from build123d import *

# Parameters (mm, degrees)
SKETCH1_W               = 13
SKETCH1_H               = 8
BOSS_EXTRUDE1_DEPTH     = 3
CUT_EXTRUDE1_DEPTH      = 16.556349186
CUT_EXTRUDE1_DEPTH_BACK = 16.556349186
CUT_EXTRUDE2_DEPTH      = 16.556349186
CUT_EXTRUDE2_DEPTH_BACK = 16.556349186
SKETCH4_R               = 1.8
CUT_EXTRUDE3_DEPTH      = 0.8
SKETCH5_W               = 8
SKETCH5_H               = 1
BOSS_EXTRUDE2_DEPTH     = 2
FILLET1_R               = 4
CUT_EXTRUDE4_DEPTH      = 0.4


with BuildPart() as part:
    # Sketch1 → Boss-Extrude1 (new body)
    with BuildSketch(Plane(origin=(0, 0, 0), x_dir=(1, 0, 0), z_dir=(0, 1, 0))):
        with Locations((6.5, 4)):
            Rectangle(SKETCH1_W, SKETCH1_H)
    extrude(amount=BOSS_EXTRUDE1_DEPTH)

    # Sketch2 → Cut-Extrude1 (cut, two sides: drawn at the far end of the back side and taken through both)
    with BuildSketch(Plane.XY.offset(-CUT_EXTRUDE1_DEPTH_BACK)):
        Polygon((0, 0), (0.6, 3), (0, 3), align=None)
        Polygon((13, 0), (12.4, 3), (13, 3), align=None)
    extrude(amount=CUT_EXTRUDE1_DEPTH + CUT_EXTRUDE1_DEPTH_BACK, mode=Mode.SUBTRACT)

    # Sketch3 → Cut-Extrude2 (cut, two sides: drawn at the far end of the back side and taken through both)
    with BuildSketch(Plane(origin=(0, 0, 0), x_dir=(0, 0, -1), z_dir=(1, 0, 0)).offset(-CUT_EXTRUDE2_DEPTH_BACK)):
        Polygon((0, 0), (0.6, 3), (0, 3), align=None)
        Polygon((8, 3), (7.4, 3), (8, 0), align=None)
    extrude(amount=CUT_EXTRUDE2_DEPTH + CUT_EXTRUDE2_DEPTH_BACK, mode=Mode.SUBTRACT)

    # Sketch4 → Cut-Extrude3 (cut)
    with BuildSketch(Plane.XZ):
        with Locations(Location((6.50000125, -3.75, 0), (0, 0, 270))):
            Circle(SKETCH4_R)
    extrude(amount=-CUT_EXTRUDE3_DEPTH, mode=Mode.SUBTRACT)

    # Sketch5 → Boss-Extrude2 (add)
    with BuildSketch(Plane.XZ):
        with Locations((6.500011, -7.5)):
            Rectangle(SKETCH5_W, SKETCH5_H)
    extrude(amount=BOSS_EXTRUDE2_DEPTH)

    # Fillet1
    # the kernel refuses this fillet: 4 mm, written as the material it takes off along each edge
    with BuildSketch(Plane(origin=(10.500011, -2, -16.660254038), x_dir=(0, 1, 0), z_dir=(0, 0, 1)), Plane(origin=(2.500011, -2, 1.660254038), x_dir=(0, 1, 0), z_dir=(0, 0, -1))) as fillet1_piece_1:
        with BuildLine():
            CenterArc((4, 3.464101615), FILLET1_R, 180, 60)
            Line((0, 3.464101615), (-0.08, 3.464101615))
            Line((-0.08, 3.464101615), (-0.08, 0))
            Line((-0.08, 0), (0, -0.08))
            ThreePointArc((0, -0.08), (1, -0.08), (1.96, -0.069282032))
            Line((1.96, -0.069282032), (2, 0))
        make_face()
    extrude(amount=18.320508076, mode=Mode.SUBTRACT)

    # Sketch6 → Cut-Extrude4 (cut)
    # profile 1 of 3: a face of its own
    with BuildSketch(Plane(origin=(0, 3, 0), x_dir=(1, 0, 0), z_dir=(0, 1, 0))):
        Polygon((5.356583629, 2.605681315), (4.744804782, 2.605681315), (4.491799975, 3.297989008), (3.340357667, 3.297989008), (3.087352859, 2.605681315), (2.471968244, 2.605681315), (3.605982667, 5.605681315), (4.217160552, 5.605681315), align=None)
        Polygon((4.308506705, 3.797989008), (3.914275936, 4.874912084), (3.52124709, 3.797989008), align=None, mode=Mode.SUBTRACT)
    # profile 2 of 3: a face of its own
    with BuildSketch(Plane(origin=(0, 3, 0), x_dir=(1, 0, 0), z_dir=(0, 1, 0))):
        Polygon((5.664275936, 2.605681315), (5.664275936, 5.605681315), (6.241199013, 5.605681315), (6.241199013, 3.105681315), (7.779660552, 3.105681315), (7.779660552, 2.605681315), align=None)
    # profile 3 of 3: a face of its own
    with BuildSketch(Plane(origin=(0, 3, 0), x_dir=(1, 0, 0), z_dir=(0, 1, 0))):
        Polygon((8.895045167, 2.605681315), (8.895045167, 5.105681315), (8.010429782, 5.105681315), (8.010429782, 5.605681315), (10.356583629, 5.605681315), (10.356583629, 5.105681315), (9.471968244, 5.105681315), (9.471968244, 2.605681315), align=None)
    extrude(amount=-CUT_EXTRUDE4_DEPTH, mode=Mode.SUBTRACT)


solid = part.part
For this review, take the finished solid that the model builds, in its own axes (mm). A direction names the side the tool comes from. Coordinates: 2 decimals unless noted, no trailing zeros. Loops run counter-clockwise (first coordinate to the right, second up) from the corner with the lowest first, then second, coordinate; pieces in that order, holes last. Notation, with made-up numbers: (67.5, 44) - (78.5, 44) arc R30 ccw to (78.5, 69) - close; hole circle Ø3 at (57.5, 20). An arc over 180 degrees is marked (long way). Return JSON: item names as keys, results as strings.
Item 1: Take a section at A-A (z = -5.25). Give the boundary of the cut face in (x, y).
Determined:
{"outline": "(0, 0) - (5.51, 0) - (5.51, 0.8) - (7.49, 0.8) - (7.49, 0) - (13, 0) - (12.4, 3) - (10.36, 3) - (10.36, 2.6) - (8.01, 2.6) - (8.01, 3) - (6.24, 3) - (6.24, 2.6) - (5.66, 2.6) - (5.66, 3) - (4.35, 3) - (4.35, 2.6) - (3.47, 2.6) - (3.47, 3) - (0.6, 3) - close"}
Item 2: For faces 1 (the flat face through (6.4, 1.5, -0.3)), 2 (the flat face through (7, 0.8, -4)), 3 (the flat face through (6, -1, -7)), 4 (the flat face through (4.779, 2.803, -4.127)), 5 (the flat face through (6.4, 1.5, -7.7)), list the 3-axis set-ups (+Z, -Z, +X, -X, +Y, -Y) from which the entire face can be reached by the end or side of a thin tool; tool diameter is ignored.
Determined:
{"face 1": "+Z, +X, -X, +Y", "face 2": "-Y", "face 3": "+Z, +X, -X, -Y", "face 4": "+Y", "face 5": "-Z, +X, -X, +Y"}
Item 3: Mouldability with a two-part tool opening along X and no side actions: class faces 6 (the flat face through (6, -1, -8)), 7 (the cylindrical face through (5.811, 0.394, -5.413)), 8 (the flat face through (0.3, 1.5, -4.1)) as pulls with the +X half, pulls with the -X half, needs draft (parallel to the pull), parting line crosses it, or undercut.
Determined:
{"face 6": "needs draft", "face 7": "undercut", "face 8": "pulls with the -X half"}
Item 4: Insertion check: pin 1 (3 mm diameter, centred on x = 8, z = -2.5, fed in from -Y); pin 2 (1.8 mm diameter, centred on x = 6, z = -4, fed in from -Y). Each pin has a flat end and moves straight along its axis. Give the tip position at first contact, or say it passes through.
Determined:
{"pin 1": "stops at y = 0", "pin 2": "stops at y = 0.8"}
Item 5: Take a section at B-B (x = 11). Give the boundary of the cut face in (y, z).
Determined:
{"outline": "(0, -8) - (3, -7.4) - (3, -0.6) - (0, 0) - close"}
Item 6: Take a section at C-C (y = -1.35). Give the boundary of the cut face in (x, z).
Determined:
{"outline": "(3.78, -8) - (9.22, -8) - (9.22, -7) - (3.78, -7) - close"}
Item 7: For line 1 (Y direction, x = 3.75, z = -0.75); line 2 (Z direction, x = 9.5, y = -0.05); line 3 (Z direction, x = 10.5, y = 0.7), list the stretches that pass through material, from the lowest coordinate up.
Determined:
{"line 1": "y = 0 to 3", "line 2": "z = -8 to -7", "line 3": "z = -7.86 to -0.14"}
Item 8: Take a section at D-D (x = 8.75). Give the boundary of the cut face in (y, z), then the cut area to 3 significant figures.
Determined:
{"outline": "(-1.61, -8) - (0, -8) - (3, -7.4) - (3, -5.61) - (2.6, -5.61) - (2.6, -5.11) - (3, -5.11) - (3, -0.6) - (0, 0) - (0, -7) - (-1.61, -7) - close", "area": "23.6 mm2"}
